Model file for the job. Use its own axes, mm. Face numbers are marked on the shaded views. A direction names the side the tool comes from. Give positions to 0.01 mm unless a question says otherwise; leave off trailing zeros. Write each loop counter-clockwise with the first axis right and the second up, starting at its lowest first coordinate (ties: lowest second). Pieces come first, ordered by that corner, then holes.
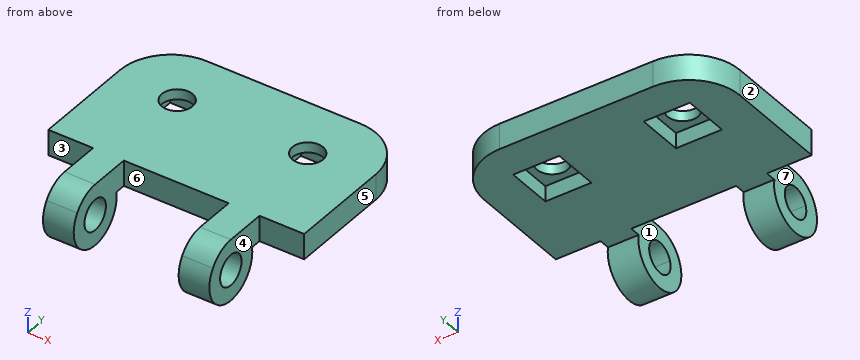
```python
from build123d import *
from build123d.topology import SkipClean

# Parameters (mm, degrees)
SALIENTE_EXTRUIR1_DEPTH    = 5
CROQUIS4_W                 = 6
CROQUIS4_H                 = 13
SALIENTE_EXTRUIR2_DEPTH    = 5
SALIENTE_EXTRUIR3_REACH    = 52.106
CROQUIS6_R                 = 6
CROQUIS6_R_2               = 3
CORTAR_EXTRUIR1_DEPTH      = 51.907391408
CORTAR_EXTRUIR1_DEPTH_BACK = 51.907391408
CORTAR_EXTRUIR2_DEPTH      = 39.923000912
CORTAR_EXTRUIR2_DEPTH_BACK = 39.923000912
CROQUIS8_W                 = 20.5
CROQUIS8_H                 = 15.513520957
CROQUIS9_R                 = 3
CORTAR_EXTRUIR3_DEPTH      = 6
CROQUIS10_W                = 9
CROQUIS10_H                = 9
CORTAR_EXTRUIR4_DEPTH      = 3


with BuildPart() as part:
    # Croquis1 → Saliente-Extruir1 (new body)
    with BuildSketch(Plane.XY):
        with BuildLine():
            Line((15, 15), (-15, 15))
            ThreePointArc((-15, 15), (-22.071067812, 12.071067812), (-25, 5))
            Line((-25, 5), (-25, -15))
            Line((-25, -15), (25, -15))
            Line((25, -15), (25, 5))
            ThreePointArc((25, 5), (22.071067812, 12.071067812), (15, 15))
        make_face()
    extrude(amount=SALIENTE_EXTRUIR1_DEPTH)

    # Croquis4 → Saliente-Extruir2 (add)
    with BuildSketch(Plane.XY.offset(5)):
        with Locations((-13.25, -21.5)):
            Rectangle(CROQUIS4_W, CROQUIS4_H)
        with Locations((13.25, -21.5)):
            Rectangle(CROQUIS4_W, CROQUIS4_H)
    extrude(amount=-SALIENTE_EXTRUIR2_DEPTH)

    # Saliente-Extruir3: up to this face of the body (flat: up to its plane)
    saliente_extruir3_end = Plane(part.part.faces().sort_by_distance((-16.25, -21.5, 2.5))[0])
    # Croquis6 → Saliente-Extruir3 (add, up to the picked face)
    with BuildSketch(Plane(origin=(16.25, 0, 0), x_dir=(0, 0, -1), z_dir=(1, 0, 0)), mode=Mode.PRIVATE) as saliente_extruir3_sk1:
        with Locations(Location((1, -23, 0), (0, 0, 99.594068227))):
            Circle(CROQUIS6_R)
        with Locations(Location((1, -23, 0), (0, 0, 109.471220634))):
            Circle(CROQUIS6_R_2, mode=Mode.SUBTRACT)
    saliente_extruir3_tool1 = split(extrude(saliente_extruir3_sk1.sketch, amount=-SALIENTE_EXTRUIR3_REACH, mode=Mode.PRIVATE), bisect_by=saliente_extruir3_end, keep=Keep.BOTH, mode=Mode.PRIVATE)
    add(saliente_extruir3_tool1.solids().sort_by(Axis((16.25, -28.748748, -1.971716), (-1, 0, 0)))[0])

    # Croquis7 → Cortar-Extruir1 (cut, two sides: drawn at the far end of the back side and taken through both)
    with SkipClean():  # the faces are left unmerged after this step: merging them gives an invalid solid
        with BuildSketch(Plane.ZY.offset(16.25).offset(-CORTAR_EXTRUIR1_DEPTH_BACK)):
            with BuildLine():
                Line((0, -20.171572875), (0, -25.828427125))
                ThreePointArc((0, -25.828427125), (-4, -23), (0, -20.171572875))
            make_face()
            with BuildLine():
                ThreePointArc((0, -25.828427125), (1.449489743, -24.732050808), (2, -23))
                ThreePointArc((2, -23), (1.449489743, -21.267949192), (0, -20.171572875))
                Line((0, -20.171572875), (0, -25.828427125))
            make_face()
            with BuildLine():
                Line((0, -25.828427125), (0, -20.171572875))
                ThreePointArc((0, -20.171572875), (-4, -23), (0, -25.828427125))
            make_face()
            with BuildLine():
                Line((5, -28), (5, -23))
                ThreePointArc((5, -23), (4.286764074, -25.837274331), (2.31662479, -28))
                Line((2.31662479, -28), (5, -28))
            make_face()
        extrude(amount=CORTAR_EXTRUIR1_DEPTH + CORTAR_EXTRUIR1_DEPTH_BACK, mode=Mode.SUBTRACT)

    # Croquis8 → Cortar-Extruir2 (cut, two sides: drawn at the far end of the back side and taken through both)
    with BuildSketch(Plane(origin=(0, 0, 0), x_dir=(-1, 0, 0), z_dir=(0, 0, -1)).offset(-CORTAR_EXTRUIR2_DEPTH_BACK)):
        with Locations((0, -22.756760479)):
            Rectangle(CROQUIS8_W, CROQUIS8_H)
    extrude(amount=CORTAR_EXTRUIR2_DEPTH + CORTAR_EXTRUIR2_DEPTH_BACK, mode=Mode.SUBTRACT)

    # Croquis9 → Cortar-Extruir3 (cut)
    with BuildSketch(Plane.XY.offset(5)):
        with Locations((-12.75, 3.5)):
            Circle(CROQUIS9_R)
        with Locations((12.75, 3.5)):
            Circle(CROQUIS9_R)
    extrude(amount=-CORTAR_EXTRUIR3_DEPTH, mode=Mode.SUBTRACT)

    # Croquis10 → Cortar-Extruir4 (cut)
    with BuildSketch(Plane(origin=(0, 0, 0), x_dir=(-1, 0, 0), z_dir=(0, 0, -1))):
        with Locations((-12.75, 3.5)):
            Rectangle(CROQUIS10_W, CROQUIS10_H)
        with Locations((12.75, 3.5)):
            Rectangle(CROQUIS10_W, CROQUIS10_H)
    extrude(amount=-CORTAR_EXTRUIR4_DEPTH, mode=Mode.SUBTRACT)


solid = part.part
```
1. Pull direction X, two halves, no side cores. Call the marked faces 1, 2 and 3: +X half, -X half, draft (parallel to the pull), parting line (faces both ways), or undercut.
Calculated:
face 1: undercut
face 2: -X half
face 3: draft
2. Slice it at A-A, the plane x = -12.75. Write the cut outline in (y, z).
Calculated:
outline: (-23, 5) arc R6 ccw (long way) to (-17.08, 0) - (-1, 0) - (-1, 3) - (0.5, 3) - (0.5, 5) - close; (6.5, 3) - (8, 3) - (8, 0) - (15, 0) - (15, 5) - (6.5, 5) - close; hole circle Ø6 at (-23, -1)
3. Slice it at C-C, the plane x = 9. Write the cut outline in (y, z).
Calculated:
outline: (-15, 0) - (-1, 0) - (-1, 3) - (8, 3) - (8, 0) - (15, 0) - (15, 5) - (-15, 5) - close
4. Pin check, flat tips, straight feed: P1, Ø0.9, axis at x = 10.5, z = 1.5, coming from the -Y side; P2, Ø2.5, axis at x = -22, z = 3.5, coming from the -Y side; P3, Ø4.5, axis at x = -13, y = 4.5, coming from the -Z side; P4, Ø6, axis at x = -8.5, z = -2.5, coming from the +Y side. Stop position of each tip, or through.
Calculated:
P1: stops at y = -28.64
P2: stops at y = -15
P3: stops at z = 3
P4: stops at y = 15
5. Slice it at B-B, the plane y = 3.5. Write the cut outline in (x, z).
Calculated:
outline: (-25, 0) - (-17.25, 0) - (-17.25, 3) - (-15.75, 3) - (-15.75, 5) - (-25, 5) - close; (-9.75, 3) - (-8.25, 3) - (-8.25, 0) - (8.25, 0) - (8.25, 3) - (9.75, 3) - (9.75, 5) - (-9.75, 5) - close; (15.75, 3) - (17.25, 3) - (17.25, 0) - (25, 0) - (25, 5) - (15.75, 5) - close
6. Slice it at D-D, the plane y = -8. Write the cut outline in (x, z).
Calculated:
outline: (-25, 0) - (25, 0) - (25, 5) - (-25, 5) - close
7. Probe probe 1 along X at (y, z) = (3.5, 1.25); probe 2 along X at (y, z) = (-24, 4.5); probe 3 along Z at (x, y) = (-13.75, -23). List the from-to ranges inside material, lowest first.
Calculated:
probe 1: x = -25 to -17.25, -8.25 to 8.25, 17.25 to 25
probe 2: x = -16.25 to -10.25, 10.25 to 16.25
probe 3: z = -7 to -4, 2 to 5
8. Which spindle directions (+Z, -Z, +X, -X, +Y, -Y) get a long thin tool onto all of the face, cutting with end or side? Do the marked faces 4, 5, 6 and 7. Say none if no direction does.
Calculated:
face 4: +Z, -Z, +X, -Y
face 5: +Z, -Z, +X, +Y, -Y
face 6: +Z, -Z, -Y
face 7: +Z, -Z, -X, -Y
